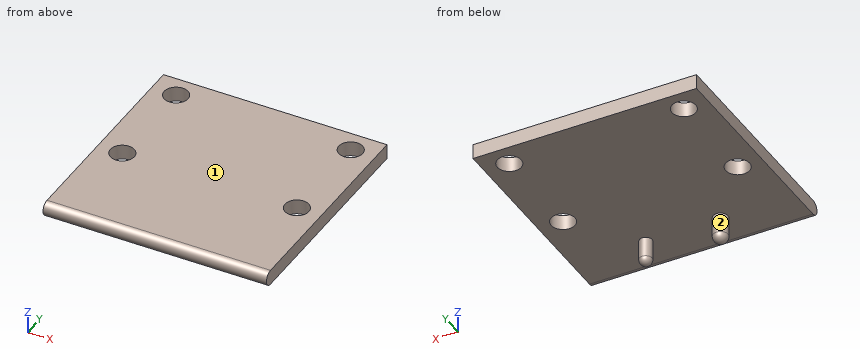
```python
from build123d import *

# Parameters (mm, degrees)
SKETCH1_W            = 44.8
SKETCH1_H            = 2.99
BOSS_EXTRUDE1_DEPTH  = 44.8
FILLET1_RADIUS       = 1.495
FILLET1_LENGTH       = 44.8
M4_CLEARANCE_HOLE1_D = 4.8
SKETCH8_R            = 1.481852537
SKETCH8_R_2          = 1.249642824
BOSS_EXTRUDE2_DEPTH  = 6.99
REVOLVE1_ANGLE       = 180
REVOLVE2_ANGLE       = 180


with BuildPart() as part:
    # Sketch1 → Boss-Extrude1 (new body)
    with BuildSketch(Plane(origin=(0, 0, 0), x_dir=(1, 0, 0), z_dir=(0, 1, 0))):
        Rectangle(SKETCH1_W, SKETCH1_H)
    extrude(amount=BOSS_EXTRUDE1_DEPTH)

    # Fillet1: full round fillet: the end face becomes a half cylinder, R = half its width
    fillet1_face = Plane((0, 0, 0), x_dir=(-1, 0, 0), z_dir=(0, -1, 0))  # on the end face: x along it, z out of the body
    fillet1_slab = fillet1_face.offset(-FILLET1_RADIUS / 2) * Box(FILLET1_LENGTH, 2 * FILLET1_RADIUS, FILLET1_RADIUS, mode=Mode.PRIVATE)  # the body's end, R deep
    fillet1_round = Plane((0, 1.495, 0), x_dir=(0, -1, 0), z_dir=(-1, 0, 0)) * Cylinder(FILLET1_RADIUS, FILLET1_LENGTH, mode=Mode.PRIVATE)  # its axis R under the face
    add(fillet1_slab - fillet1_round, mode=Mode.SUBTRACT)

    # M4 Clearance Hole1 (through all)
    with Locations(Plane.XY.offset(1.495)):
        with Locations((-17.5, 40.4), (-17.5, 20.4), (17.5, 20.4), (17.5, 40.4)):
            Hole(M4_CLEARANCE_HOLE1_D / 2)

    # Sketch8 → Boss-Extrude2 (add)
    with BuildSketch(Plane.XY.offset(1.495)):
        with Locations((-7.5, 8.2)):
            Circle(SKETCH8_R)
        with Locations((7.5, 8.2)):
            Circle(SKETCH8_R_2)
    extrude(amount=-BOSS_EXTRUDE2_DEPTH)

    # Sketch9 → Revolve1 (revolve)
    with BuildSketch(Plane(origin=(0, 0, -5.495), x_dir=(-1, 0, 0), z_dir=(0, 0, -1))):
        with BuildLine():
            Line((7.5, 9.681852537), (7.5, 6.718147463))
            ThreePointArc((7.5, 6.718147463), (8.981852537, 8.2), (7.5, 9.681852537))
        make_face()
    revolve(axis=Axis((-7.5, 9.681852537, -5.495), (0, -1, 0)), revolution_arc=REVOLVE1_ANGLE)

    # Sketch10 → Revolve2 (revolve)
    with BuildSketch(Plane(origin=(0, 0, -5.495), x_dir=(-1, 0, 0), z_dir=(0, 0, -1))):
        with BuildLine():
            Line((-7.5, 9.449642824), (-7.5, 6.950357176))
            ThreePointArc((-7.5, 6.950357176), (-6.250357176, 8.2), (-7.5, 9.449642824))
        make_face()
    revolve(axis=Axis((7.5, 9.449642824, -5.495), (0, -1, 0)), revolution_arc=REVOLVE2_ANGLE)


solid = part.part
```
The listing builds one solid part. Answer for the finished solid, in the listing's coordinates (mm). Face numbers are marked on the shaded views. Coordinates: 2 decimals unless noted, no trailing zeros. Loops run counter-clockwise (first coordinate to the right, second up) from the corner with the lowest first, then second, coordinate; pieces in that order, holes last. Notation, with made-up numbers: M 34,33 L 52,33 A26 cw 52,56 Z; hole C 16,1.25 d4. An arc over 180 degrees is marked long. Answer as CSV lines item,"result". Start each with the question number.
(1) Find the intervals of material crossed by L1, parallel to Y at x = -17.5, z = -0.2; L2, parallel to Y at x = -19, z = 0.25; L3, parallel to Z at x = -12, y = 14 (3 decimals), in increasing order. Write a range as [from, to].
(2) The part is cut by section A-A (x = 17.5). Give the vertices of the cut face in (y, z) (3 decimals).
(3) Given pin 1 (21.5 mm diameter, centred on x = 9, y = 13.5, fed in from -Z); pin 2 (6 mm diameter, centred on x = -17.5, y = 40.4, fed in from -Z) (3 decimals); pin 3 (4 mm diameter, centred on x = 17.5, y = 20.4, fed in from +Z), each flat-ended and moving along its own axis, determine where each tip first touches the part or whether it passes through.
(4) The mould has two halves that part along X. Classify the marked faces 1 and 2: pulls with the +X half, pulls with the -X half, needs draft (parallel to the pull), parting line crosses it, or undercut.
(5) The part is cut by section C-C (z = 0). Give the vertices of the cut face in (x, y).
(6) The part is cut by section D-D (z = -3.5). Give the vertices of the cut face in (x, y).
(7) The part is cut by section B-B (y = 20.4). Give the vertices of the cut face in (x, z) (3 decimals).
Determined:
1,L1,"[0.01, 18], [22.8, 38], [42.8, 44.8]"
1,L2,"[0.02, 18.53], [22.27, 38.53], [42.27, 44.8]"
1,L3,"[-1.495, 1.495]"
2,outline,"M 1.495,-1.495 L 18,-1.495 L 18,1.495 L 1.495,1.495 A1.495 ccw Z; M 22.8,-1.495 L 38,-1.495 L 38,1.495 L 22.8,1.495 Z; M 42.8,-1.495 L 44.8,-1.495 L 44.8,1.495 L 42.8,1.495 Z"
3,pin 1,"z = -6.74"
3,pin 2,"z = -1.495"
3,pin 3,"through"
4,face 1,"needs draft"
4,face 2,"undercut"
5,outline,"M -22.4,0 L 22.4,0 L 22.4,44.8 L -22.4,44.8 Z; hole C -17.5,20.4 d4.8; hole C -17.5,40.4 d4.8; hole C 17.5,20.4 d4.8; hole C 17.5,40.4 d4.8"
6,outline,"C -7.5,8.2 d2.96; C 7.5,8.2 d2.5"
7,outline,"M -22.4,-1.495 L -19.9,-1.495 L -19.9,1.495 L -22.4,1.495 Z; M -15.1,-1.495 L 15.1,-1.495 L 15.1,1.495 L -15.1,1.495 Z; M 19.9,-1.495 L 22.4,-1.495 L 22.4,1.495 L 19.9,1.495 Z"
